Check sheet for the drawn part. Datum: minimum x, y, z corner. Units: mm. Give positions to 0.01 mm unless a question says otherwise; leave off trailing zeros. Order: outer loops, then holes, each group sorted by start corner. A loop starts at its lowest first (then second) coordinate and runs counter-clockwise, first axis right, second up. Notation, with made-up numbers: M -23.5,47 L -12.5,47 A24 ccw -12.5,67 Z; hole C 57,-32 d10. An arc over 180 degrees is marked long. Answer as CSV lines item,"result". Start each with the question number.
Q1. Section check A-A, the plane z = 107.95. Record the boundary of the cut face in (x, y) (3 decimals).
Q2. Thickness scan on line 1 (Z direction, x = 1, y = 63.5); line 2 (Y direction, x = 0.95, z = 82.55); line 3 (Y direction, x = 1.7, z = 107.95). Record the ranges inside material, lowest first.
Q3. Section check B-B, the plane y = 25.4. Record the boundary of the cut face in (x, z) (3 decimals), then the cut area to 3 significant figures.
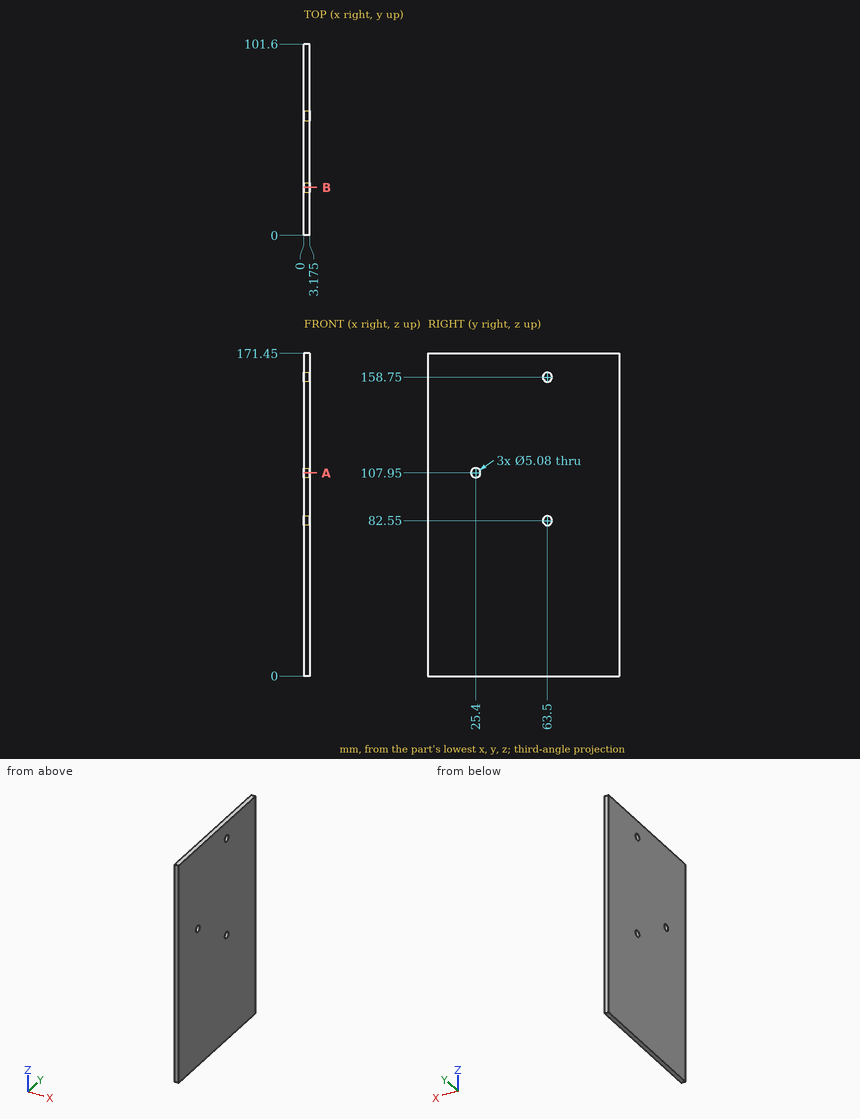
Answer block:
1,outline,"M 0,0 L 3.175,0 L 3.175,22.86 L 0,22.86 Z; M 0,27.94 L 3.175,27.94 L 3.175,101.6 L 0,101.6 Z"
2,line 1,"z = 0 to 80.01, 85.09 to 156.21, 161.29 to 171.45"
2,line 2,"y = 0 to 60.96, 66.04 to 101.6"
2,line 3,"y = 0 to 22.86, 27.94 to 101.6"
3,outline,"M 0,0 L 3.175,0 L 3.175,105.41 L 0,105.41 Z; M 0,110.49 L 3.175,110.49 L 3.175,171.45 L 0,171.45 Z"
3,area,"528 mm2"
